Design review of the part built by this model. Coordinates are the model's own, in mm. A direction names the side the tool comes from. Give positions to 0.01 mm unless a question says otherwise; leave off trailing zeros. Order: outer loops, then holes, each group sorted by start corner. A loop starts at its lowest first (then second) coordinate and runs counter-clockwise, first axis right, second up. Notation, with made-up numbers: (17.5, -20.5) -> (63.5, -20.5) arc R12 cw to (63.5, -11.5) -> close; hole circle Ø5 at (-11, -25). An arc over 180 degrees is marked (long way). One line per item, written item: value.
Autodesk Inventor part; units mm, degrees
ref_plane "YZ Plane" through (0, 0, 0) normal (1, 0, 0) x (0, 1, 0)
ref_plane "XZ Plane" through (0, 0, 0) normal (0, 1, 0) x (-1, 0, 0)
ref_plane "XY Plane" through (0, 0, 0) normal (0, 0, 1) x (1, 0, 0)
sketch "Sketch1" plane through (0, 0, 0) normal (0, 0, 1) x (1, 0, 0)
  line L0 (0, 0) -> (25.4, 0)
  line L1 (25.4, 0) -> (25.4, 76.2)
  line L2 (25.4, 76.2) -> (0, 76.2)
  line L3 (0, 76.2) -> (0, 0)
  line L4 (3.175, 3.175) -> (22.225, 3.175)
  line L5 (22.225, 3.175) -> (22.225, 73.025)
  line L6 (22.225, 73.025) -> (3.175, 73.025)
  line L7 (3.175, 73.025) -> (3.175, 3.175)
  dimension "d0" = 25.4
  dimension "d1" = 76.2
  dimension "d2" = 3.175
  dimension "d3" = 3.175
  dimension "d4" = 3.175
  dimension "d5" = 3.175
extrude "Extrusion1" add sketch "Sketch1" along normal blind 679.45
sketch "Sketch2" plane through (0, 76.2, 0) normal (0, 1, 0) x (1, 0, 0)
  line L0 (0, -679.45) -> (25.4, -679.45)
  line L1 (25.4, 0) -> (25.4, -679.45)
  line L2 (25.4, 0) -> (0, 0)
  line L3 (0, 0) -> (0, -679.45)
  line L4 (0, -22.225) -> (25.4, -22.225)
  line L5 (0, -657.225) -> (25.4, -657.225)
  dimension "d8" = 22.225
  dimension "d9" = 22.225
extrude "Extrusion2" cut sketch "Sketch2" against normal blind 3.175 contours L3 L5 L1 L0 | L3 L2 L1 L4
sketch "Sketch3" plane through (0, 0, 0) normal (0, -1, 0) x (1, 0, 0)
  line L0 (25.4, 679.45) -> (0, 679.45)
  line L1 (0, 0) -> (0, 679.45)
  line L2 (0, 0) -> (25.4, 0)
  line L3 (25.4, 0) -> (25.4, 679.45)
  line L4 (0, 657.225) -> (25.4, 657.225)
  line L5 (0, 22.225) -> (25.4, 22.225)
  dimension "d12" = 22.225
  dimension "d13" = 22.225
extrude "Extrusion3" cut sketch "Sketch3" against normal blind 3.175 contours L3 L4 L1 L0 | L3 L2 L1 L5
equation "\"d3\" = d2"
equation "\"d4\" = d3"
equation "\"d5\" = d4"
equation "\"d9\" = d8"
equation "\"d13\" = d12"
properties part number "frame box 1 by 3"
Item 1: Add section A-A on x = 9.75. Give the boundary of the cut face in (y, z) (3 decimals).
Returned:
outline: (0, 22.225) -> (3.175, 22.225) -> (3.175, 657.225) -> (0, 657.225) -> close; (73.025, 22.225) -> (76.2, 22.225) -> (76.2, 657.225) -> (73.025, 657.225) -> close
Item 2: Add section C-C on y = 20. Give the boundary of the cut face in (x, z) (3 decimals).
Returned:
outline: (0, 0) -> (3.175, 0) -> (3.175, 679.45) -> (0, 679.45) -> close; (22.225, 0) -> (25.4, 0) -> (25.4, 679.45) -> (22.225, 679.45) -> close
Item 3: To check wall thickness, follow line 1 along X through (y, z) = (11, 40.5) (3 decimals); line 2 along Y through (x, z) = (14.25, 560) (3 decimals); line 3 along Z through (x, y) = (7.5, 3) (3 decimals). State the ranges of each line that lie inside material, in increasing order. Write a range as from..to.
Returned:
line 1: 0..3.175, 22.225..25.4
line 2: 0..3.175, 73.025..76.2
line 3: 22.225..657.225
Item 4: Machinability: for faces 1 (the flat face through (3.175, 39, 335)), 2 (the flat face through (25.4, 38, 335)), which of the approach directions +Z, -Z, +X, -X, +Y, -Y give a long, thin tool a straight path to every point of the face, cutting with its end or side? Answer none if there is none.
Returned:
face 1: +Z, -Z
face 2: +Z, -Z, +X, +Y, -Y
Item 5: Add section B-B on z = 57. Give the boundary of the cut face in (x, y) (3 decimals).
Returned:
outline: (0, 0) -> (25.4, 0) -> (25.4, 76.2) -> (0, 76.2) -> close; hole (3.175, 3.175) -> (22.225, 3.175) -> (22.225, 73.025) -> (3.175, 73.025) -> close
Item 6: Clearance check with flat-ended pins moving along their axes: P1, Ø3.5, axis at x = 24, z = 664, coming from the -Y side (3 decimals); P2, Ø1.6, axis at x = 15.5, y = 2, coming from the -Z side (3 decimals); P3, Ø2.5, axis at x = 1, z = 14, coming from the +Y side (3 decimals); P4, Ø8, axis at x = 9, y = 35, coming from the +Z side. State where each tip first meets the part, or that it passes through.
Returned:
P1: y = 3.175
P2: z = 22.225
P3: y = 73.025
P4: through
Item 7: Draft analysis for pull direction Y (two halves, no side actions). For faces 3 (the flat face through (13, 0, 335)), 4 (the flat face through (13, 76.2, 335)), 5 (the flat face through (13, 73.025, 335)), state which applies: pulls with the +Y half, pulls with the -Y half, needs draft (parallel to the pull), parting line crosses it, or undercut.
Returned:
face 3: pulls with the -Y half
face 4: pulls with the +Y half
face 5: undercut
